Can you work these out from the drawing? Everything is in mm from the part's minimum corner. Round coordinates to 2 decimals unless told otherwise and drop trailing zeros. Loops run counter-clockwise (first coordinate to the right, second up) from the corner with the lowest first, then second, coordinate; pieces in that order, holes last. Notation, with made-up numbers: M -36.5,-38.5 L -28.5,-38.5 A29 ccw -28.5,-3.5 Z; hole C 49.25,-11.5 d2. An arc over 180 degrees is marked long. Answer in a Markdown table with one row per item.
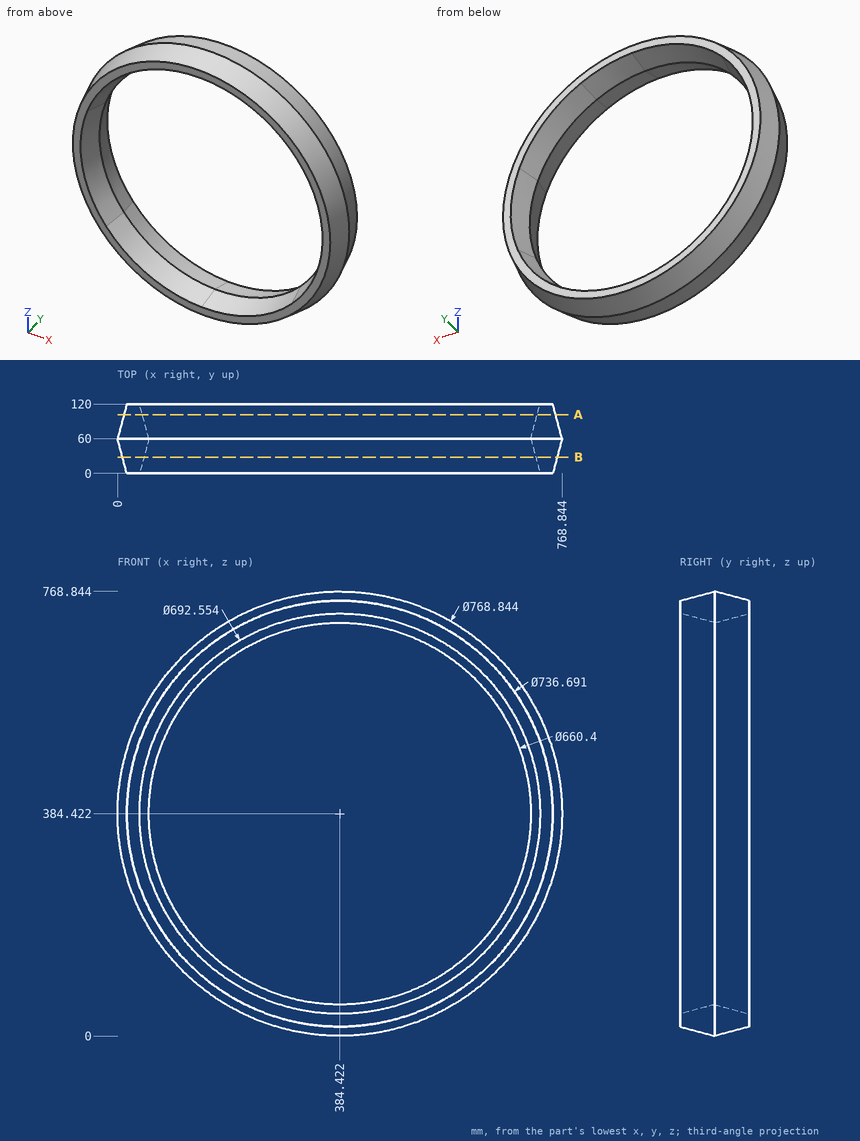
1) Will these pins go through, and if not, where does the flat tip stop? P1, Ø10, axis at y = 56, z = 355, coming from the -X side; P2, Ø1.5, axis at x = 230.5, y = 100, coming from the +Z side; P3, Ø5, axis at x = 623, y = 90, coming from the -Z side (1 decimal).
Computed:
| item | result |
|---|---|
| P1 | stops at x = 0.91 |
| P2 | stops at z = 725.36 |
| P3 | stops at z = 91.1 |
2) I want a section at B-B, the plane y = 28. Please give me the cut outline in (x, z) (1 decimal).
Computed:
| item | result |
|---|---|
| outline | C 384.4,384.4 d751.7; hole C 384.4,384.4 d677.5 |
3) I need wall thicknesses on line 1 (X direction, y = 38, z = 377.5) (1 decimal); line 2 (Z direction, x = 134, y = 53) (1 decimal); line 3 (X direction, y = 61.5, z = 440) (1 decimal). Which ranges of each line are inside material? Lowest first, please.
Computed:
| item | result |
|---|---|
| line 1 | x = 6 to 48.4, 720.4 to 762.9 |
| line 2 | z = 95.2 to 166.3, 602.5 to 673.6 |
| line 3 | x = 4.4 to 58.5, 710.3 to 764.4 |
4) I want a section at A-A, the plane y = 101.5. Please give me the cut outline in (x, z) (1 decimal).
Computed:
| item | result |
|---|---|
| outline | C 384.4,384.4 d746.6; hole C 384.4,384.4 d682.6 |
